CAD build for the part. Positions are in the model's coordinates, mm. A direction names the side the tool comes from. Round coordinates to 2 decimals unless told otherwise and drop trailing zeros. Order: outer loops, then holes, each group sorted by start corner. A loop starts at its lowest first (then second) coordinate and runs counter-clockwise, first axis right, second up.
```python
from build123d import *

# Parameters (mm, degrees)
F0_W     = 19.05
F0_H     = 19.05
F0_R     = 3.96875
F1_DEPTH = 6.35
F6_DEPTH = 19.051


with BuildPart() as f1:
    # F0 (on Top) → F1 (new body)
    with BuildSketch(Plane.XY):
        Rectangle(F0_W, F0_H)
        Circle(F0_R, mode=Mode.SUBTRACT)
    extrude(amount=F1_DEPTH)

    # F4: sweep along a path in F2
    with BuildLine(Plane(origin=(0, 0, 0), x_dir=(1, 0, 0), z_dir=(0, 0, -1))) as f4_path:
        CenterArc((0, 0), 9.525, 0, 360)
    # F3 (on Right) → F4 (sweep, cut)
    with BuildSketch(Plane.YZ):
        Polygon((-20.809421, 0), (-9.525, 0), (-20.809421, 3.023652), align=None)
    sweep(path=f4_path.line, mode=Mode.SUBTRACT)

    # F5 (on face) → F6 (cut, through all)
    with BuildSketch(Plane(origin=(-9.525, 0, 0), x_dir=(0, -1, 0), z_dir=(-1, 0, 0))):
        Polygon((-7.59023, 6.35), (-9.525, 6.35), (-9.525, 4.41523), align=None)
    extrude(amount=-F6_DEPTH, mode=Mode.SUBTRACT)

    # F7: F1 across face


with BuildPart() as f1_1:
    add(f1.part)
    add(f1.part.mirror(Plane(origin=(0, -1.140472, 6.35), x_dir=(1, 0, 0), z_dir=(0, 0, 1))))


solid = f1_1.part
```
1. Cut at B-B, the plane z = 7.25. Write the cut outline in (x, y) (1 decimal), and give its area (3 significant figures).
2. Cut at A-A, the plane z = 10.5. Write the cut outline in (x, y) (1 decimal).
3. Pin check, flat tip, straight feed: P1, Ø7, axis at x = 0, y = 0, coming from the +Z side. Stop position of the tip, or through.
4. Tool access for faces 5 (the face through (-0.13, 8.57, 5.37)), 6 (the face through (-7.386, -7.44, 0.257)): list every direction of +Z, -Z, +X, -X, +Y, -Y with a clear straight run to the whole face (end or side of a thin tool).
5. Drill centre lines: line 1 (Y direction, x = -1.5, z = 8.25) (3 decimals); line 2 (Y direction, x = 2.5, z = 4) (3 decimals); line 3 (X direction, y = 1.75, z = 10) (3 decimals). Where is each one in solid material? Low to high.
6. Mould opens along Z. For faces 1 (the face through (0, 9.525, 2)), 2 (the face through (-7.44, 7.386, 0.257)), 3 (the face through (-0.13, 8.57, 7.33)), 4 (the face through (7.386, 7.44, 12.443)) say: released by +Z, released by -Z, zero draft, split by the parting line, or undercut.
Outcome:
1. outline: (-9.5, -9.5) - (9.5, -9.5) - (9.5, 8.5) - (-9.5, 8.5) - close; hole circle Ø7.9 at (0, 0)
1. area: 294 mm2
2. outline: (-9.5, -9.5) - (9.5, -9.5) - (9.5, 9.5) - (-9.5, 9.5) - close; hole circle Ø7.9 at (0, 0)
3. P1: passes through
4. face 5: +X, -X, +Y
4. face 6: -Z, -X, -Y
5. line 1: y = -9.525 to -3.674, 3.674 to 9.49
5. line 2: y = -9.525 to -3.082, 3.082 to 9.525
5. line 3: x = -9.525 to -3.562, 3.562 to 9.525
6. face 1: zero draft
6. face 2: released by -Z
6. face 3: undercut
6. face 4: released by +Z
